Verification items for the finished model (mm, model axes). A direction names the side the tool comes from. Coordinates: 2 decimals unless noted, no trailing zeros. Order: outer loops, then holes, each group sorted by start corner. A loop starts at its lowest first (then second) coordinate and runs counter-clockwise, first axis right, second up. Notation, with made-up numbers: M 86,17 L 123,17 A15 cw 123,43 Z; hole C -15,20 d2. An arc over 180 degrees is marked long. Answer as a JSON object with one key per item and string values. Group by question number.
(1) Cross-section at A-A (z = 25.5). Enter the section's corners in (x, y), plus the area to 3 significant figures.
(2) Gauge pin test, flat end, axial feed: pin 1 Ø3 at (x, z) = (-15, -8.5) entering from +Y. Record the tip position at first contact, or that the pin passes through.
(3) Mould release check, pull along Z, two halves, no side actions. Record for faces 4 (the face through (-8.38, 0.81, -11.82)), 5 (the face through (11.82, 0.81, 8.38)), 6 (the face through (2.83, 0.79, 18.55)): released by +Z, released by -Z, zero draft, split by the parting line, or undercut.
(4) Access from +Z, -Z, +X, -X, +Y, -Y to the whole of each face (thin tool, end or side, straight path). Record for faces 1 (the face through (20.59, 0.79, 19.15)), 2 (the face through (-19.15, 0.79, 20.59)), 3 (the face through (-18.55, 0.79, 2.83)).
(5) Cross-section at B-B (x = -19.5). Enter the section's corners in (y, z), plus the area to 3 significant figures.
(6) Material ranges on line 1 (X direction, y = 0.95, z = -13.5); line 2 (X direction, y = 1.1, z = -18.5); line 3 (Z direction, x = -23, y = 0.5), recorded low to high.
(7) Cross-section at C-C (z = -19.5). Enter the section's corners in (x, y).
(8) Cross-section at D-D (x = 3). Enter the section's corners in (y, z), plus the area to 3 significant figures.
from build123d import *

# Parameters (mm, degrees)
BOSS_EXTRUDE1_DEPTH = 1.6
FILLET1_R           = 1.016
FILLET3_R           = 3.81


with BuildPart() as part:
    # Framesketch → Boss-Extrude1 (new body)
    with BuildSketch(Plane(origin=(0, 0, 0), x_dir=(1, 0, 0), z_dir=(0, 1, 0))):
        with BuildLine():
            Line((-27.040136119, 28.482633953), (-8.475620882, 9.918118716))
            ThreePointArc((-8.475620882, 9.918118716), (-3.768551726, 16.575119627), (-1.023018488, 24.251981512))
            Line((-1.023018488, 24.251981512), (0, 25.275))
            Line((0, 25.275), (1.023018488, 24.251981512))
            ThreePointArc((1.023018488, 24.251981512), (3.768551726, 16.575119627), (8.475620882, 9.918118716))
            Line((8.475620882, 9.918118716), (27.040136119, 28.482633953))
            Line((27.040136119, 28.482633953), (28.482633953, 27.040136119))
            Line((28.482633953, 27.040136119), (9.918118716, 8.475620882))
            ThreePointArc((9.918118716, 8.475620882), (16.575119627, 3.768551726), (24.251981512, 1.023018488))
            Line((24.251981512, 1.023018488), (25.275, 0))
            Line((25.275, 0), (24.251981512, -1.023018488))
            ThreePointArc((24.251981512, -1.023018488), (16.575119627, -3.768551726), (9.918118716, -8.475620882))
            Line((9.918118716, -8.475620882), (28.482633953, -27.040136119))
            Line((28.482633953, -27.040136119), (27.040136119, -28.482633953))
            Line((27.040136119, -28.482633953), (8.475620882, -9.918118716))
            ThreePointArc((8.475620882, -9.918118716), (3.768551726, -16.575119627), (1.023018488, -24.251981512))
            Line((1.023018488, -24.251981512), (0, -25.275))
            Line((0, -25.275), (-1.023018488, -24.251981512))
            ThreePointArc((-1.023018488, -24.251981512), (-3.768551726, -16.575119627), (-8.475620882, -9.918118716))
            Line((-8.475620882, -9.918118716), (-27.040136119, -28.482633953))
            Line((-27.040136119, -28.482633953), (-28.482633953, -27.040136119))
            Line((-28.482633953, -27.040136119), (-9.918118716, -8.475620882))
            ThreePointArc((-9.918118716, -8.475620882), (-16.575119627, -3.768551726), (-24.251981512, -1.023018488))
            Line((-24.251981512, -1.023018488), (-25.275, 0))
            Line((-25.275, 0), (-24.251981512, 1.023018488))
            ThreePointArc((-24.251981512, 1.023018488), (-16.575119627, 3.768551726), (-9.918118716, 8.475620882))
            Line((-9.918118716, 8.475620882), (-28.482633953, 27.040136119))
            Line((-28.482633953, 27.040136119), (-27.040136119, 28.482633953))
        make_face()
    extrude(amount=BOSS_EXTRUDE1_DEPTH)

    # Fillet1
    fillet1_edges = [part.edges().sort_by_distance(p)[0] for p in [
        (-25.275, 0.8, 0),
        (0, 0.8, -25.275),
        (25.275, 0.8, 0),
        (0, 0.8, 25.275),
    ]]
    fillet(fillet1_edges, radius=FILLET1_R)

    # Fillet3
    fillet3_edges = [part.edges().sort_by_distance(p)[0] for p in [
        (-8.475620882, 0.8, 9.918118716),
        (-9.918118716, 0.8, 8.475620882),
        (-9.918118716, 0.8, -8.475620882),
        (-8.475620882, 0.8, -9.918118716),
        (8.475620882, 0.8, -9.918118716),
        (9.918118716, 0.8, -8.475620882),
        (9.918118716, 0.8, 8.475620882),
        (8.475620882, 0.8, 9.918118716),
    ]]
    fillet(fillet3_edges, radius=FILLET3_R)


solid = part.part
Taken from the geometry:
{
 "1": {"outline": "M -26.94,0 L -24.06,0 L -24.06,1.6 L -26.94,1.6 Z; M 24.06,0 L 26.94,0 L 26.94,1.6 L 24.06,1.6 Z", "area": "9.23 mm²"},
 "2": {"pin 1": "passes through"},
 "3": {"face 4": "released by -Z", "face 5": "undercut", "face 6": "released by +Z"},
 "4": {"face 1": "+X, +Y, -Y", "face 2": "+Z, +Y, -Y", "face 3": "-X, +Y, -Y"},
 "5": {"outline": "M 0,-20.94 L 1.6,-20.94 L 1.6,-18.06 L 0,-18.06 Z; M 0,-2.44 L 1.6,-2.44 L 1.6,2.44 L 0,2.44 Z; M 0,18.06 L 1.6,18.06 L 1.6,20.94 L 0,20.94 Z", "area": "17.0 mm²"},
 "6": {"line 1": "x = -14.94 to -12.06, -5.61 to 5.61, 12.06 to 14.94", "line 2": "x = -19.94 to -17.06, -2.85 to 2.85, 17.06 to 19.94", "line 3": "z = -24.44 to -21.56, -1.31 to 1.31, 21.56 to 24.44"},
 "7": {"outline": "M -20.94,0 L -18.06,0 L -18.06,1.6 L -20.94,1.6 Z; M -2.44,0 L 2.44,0 L 2.44,1.6 L -2.44,1.6 Z; M 18.06,0 L 20.94,0 L 20.94,1.6 L 18.06,1.6 Z"},
 "8": {"outline": "M 0,-18.17 L 1.6,-18.17 L 1.6,18.17 L 0,18.17 Z", "area": "58.1 mm²"}
}
